Build history of the part. All positions in model axes, mm. Face numbers are marked on the shaded views. A direction names the side the tool comes from. Give positions to 0.01 mm unless a question says otherwise; leave off trailing zeros. Write each loop counter-clockwise with the first axis right and the second up, starting at its lowest first coordinate (ties: lowest second). Pieces come first, ordered by that corner, then holes. Notation, with made-up numbers: M -2,51 L 53,51 A5 cw 53,56 Z; hole C -32.75,86.25 d6. An arc over 180 degrees is marked long. Return JSON: item names as keys, results as strings. Group by question number.
Q1. Tool access for the marked faces 1, 2 and 3: list every direction of +Z, -Z, +X, -X, +Y, -Y with a clear straight run to the whole face (end or side of a thin tool).
Q2. Band-saw the part on A-A, the plane y = 4.5. Give the cut face in (x, z), then the cut area to 3 significant figures.
Q3. Pull direction X, two halves, no side cores. Call the marked faces 4, 5 and 6: +X half, -X half, draft (parallel to the pull), parting line (faces both ways), or undercut.
Q4. Flat gauge pins, fed straight in: pin 1 Ø6 at (y, z) = (12, 17) entering from +X; pin 2 Ø5 at (x, z) = (13.5, 12.5) entering from +Y; pin 3 Ø4.5 at (x, y) = (2, 10) entering from +Z. Where does each tip first touch, or does it go through?
Q5. Wall check: probe 1 along X at (y, z) = (4.5, 12); probe 2 along Z at (x, y) = (12, 2.65). Give the ranges that are in metal, low to high.
Q6. Band-saw the part on D-D, the plane x = 27. Give the cut face in (y, z), then the cut area to 3 significant figures.
Q7. Band-saw the part on B-B, the plane x = 12. Give the cut face in (y, z).
Q8. Band-saw the part on C-C, the plane z = 12. Give the cut face in (x, y).
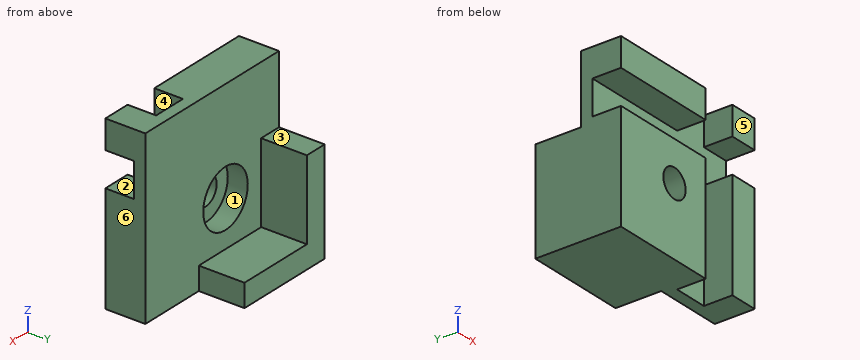
Autodesk Fusion 360 part; units mm, degrees
sketch "Sketch1" plane through (0, 0, 0) normal (0, 1, 0) x (1, 0, 0)
  line L0 (0, 0) -> (30, 0)
  line L1 (30, 0) -> (30, -30)
  line L2 (30, -30) -> (0, -30)
  line L3 (0, -30) -> (0, 0)
  dimension "d1" = 30
  dimension "d2" = 30
extrude "Extrude1" add sketch "Sketch1" along normal blind 7
sketch "Sketch2" plane through (0, 7, 0) normal (0, 1, 0) x (-1, 0, 0)
  line L0 (0, 30) -> (-30, 30)
  line L1 (-30, 30) -> (-30, 0)
  line L2 (-18, 0) -> (-18, 4)
  line L3 (-18, 4) -> (-4, 4)
  line L4 (-4, 4) -> (-4, 18)
  line L5 (-4, 18) -> (0, 18)
  line L6 (0, 18) -> (0, 0)
  line L7 (0, 0) -> (-18, 0)
  dimension "d9" = 18
  dimension "d10" = 18
  dimension "d11" = 4
  dimension "d12" = 4
extrude "Extrude2" add sketch "Sketch2" along normal blind 8
sketch "Sketch3" plane through (0, 0, 0) normal (0, 0, -1) x (-1, 0, 0)
  line L0 (-30, 0) -> (0, 0)
  line L1 (0, 0) -> (0, 15)
  line L2 (0, 15) -> (-18, 15)
  line L3 (-18, 15) -> (-18, 7)
  line L4 (-18, 7) -> (-30, 7)
  line L5 (-30, 7) -> (-30, 0)
  line L6 (-25, 0) -> (-19, 0)
  line L7 (-19, 0) -> (-19, 5)
  line L8 (-19, 5) -> (-25, 5)
  line L9 (-25, 5) -> (-25, 0)
  dimension "d13" = 6
  dimension "d14" = 5
  dimension "d15" = 5
extrude "Extrude3" cut sketch "Sketch3" against normal through all contours L0 L6 L7 L8 L9
sketch "Sketch4" plane through (0, 7, 0) normal (0, 1, 0) x (-1, 0, 0)
  line L0 (-4, 18) -> (0, 18)
  line L1 (0, 18) -> (0, 30)
  line L2 (0, 30) -> (-30, 30)
  line L3 (-30, 30) -> (-30, 0)
  line L4 (-30, 0) -> (-18, 0)
  line L5 (-18, 0) -> (-18, 4)
  line L6 (-18, 4) -> (-4, 4)
  line L7 (-4, 4) -> (-4, 18)
  line L8 (-19, 0) -> (-19, 30)
  point P0 (-12, 12)
  dimension "d18" = 8
  dimension "d28" = 8
hole "Hole1" at (12, 7, 12) direction (0, -1, 0) diameter 5 end through all counterbore diameter 10 counterbore depth 3.5
sketch "Sketch5" plane through (0, 0, 0) normal (-1, 0, 0) x (0, 0, 1)
  line L0 (0, 0) -> (30, 0)
  line L1 (30, 0) -> (30, 7)
  line L2 (30, 7) -> (18, 7)
  line L3 (18, 7) -> (18, 15)
  line L4 (18, 15) -> (0, 15)
  line L5 (0, 15) -> (0, 0)
  line L6 (25, 0) -> (19, 0)
  line L7 (19, 0) -> (19, 5)
  line L8 (19, 5) -> (25, 5)
  line L9 (25, 5) -> (25, 0)
  dimension "d24" = 6
  dimension "d25" = 5
  dimension "d26" = 5
extrude "Extrude4" cut sketch "Sketch5" against normal through all contours L0 L6 L7 L8 L9
equation "d9 = d10"
From the geometry:
{
 "1": {"face 1": "+Y", "face 2": "+X, -X, -Y", "face 3": "+Z, +X, -X, +Y"},
 "2": {"outline": "M 0,0 L 19,0 L 19,19 L 0,19 Z; M 0,25 L 19,25 L 19,30 L 0,30 Z; M 25,0 L 30,0 L 30,19 L 25,19 Z; M 25,25 L 30,25 L 30,30 L 25,30 Z; hole C 12,12 d10", "area": "497 mm^2"},
 "3": {"face 4": "undercut", "face 5": "draft", "face 6": "+X half"},
 "4": {"pin 1": "stops at x = 4", "pin 2": "stops at y = 3.5", "pin 3": "stops at z = 18"},
 "5": {"probe 1": "x = 0 to 7, 17 to 19, 25 to 30", "probe 2": "z = 0 to 9.5, 14.5 to 19, 25 to 30"},
 "6": {"outline": "M 0,0 L 7,0 L 7,30 L 0,30 L 0,25 L 5,25 L 5,19 L 0,19 Z", "area": "180 mm^2"},
 "7": {"outline": "M 0,0 L 15,0 L 15,4 L 7,4 L 7,7 L 3.5,7 L 3.5,9.5 L 0,9.5 Z; M 0,14.5 L 3.5,14.5 L 3.5,17 L 7,17 L 7,30 L 0,30 L 0,25 L 5,25 L 5,19 L 0,19 Z"},
 "8": {"outline": "M 0,0 L 9.5,0 L 9.5,3.5 L 7,3.5 L 7,7 L 4,7 L 4,15 L 0,15 Z; M 14.5,0 L 19,0 L 19,5 L 25,5 L 25,0 L 30,0 L 30,7 L 17,7 L 17,3.5 L 14.5,3.5 Z"}
}
